Autodesk Inventor part; units mm, degrees
ref_plane "Work Plane1" through (-14.5, -35, 0) normal (0, -1, 0) x (1, 0, 0)
ref_plane "Work Plane4" through (-14.5, -35, 0) normal (-1, 0, 0) x (0, 0, 1)
ref_plane "YZ Plane" through (0, 0, 0) normal (1, 0, 0) x (0, 1, 0)
ref_plane "Work Plane1" through (-14.5, -35, 0) normal (0, -1, 0) x (1, 0, 0)
sketch "Sketch2" plane through (-14.5, -35, 0) normal (0, -1, 0) x (1, 0, 0)
  line L0 (4.3469, 0) -> (4.3469, 20)
  line L1 (7.596, 20) -> (7.4184, 20)
  line L2 (4.3469, 20) -> (7.596, 20)
  arc A0 (7.596, 20) -> (29, 8.6937) centre (18.17, 14.1045) ccw
  line L3 (4.3469, 0) -> (18.3998, 0)
  arc A1 (18.3998, 0) -> (29, 8.6937) centre (18.9461, 10.1431) ccw
  point P0 (14.5, 0)
  point P1 (5, 0)
  point P2 (18.2531, 1.9984)
extrude "Extrusion1" add sketch "Sketch2" against normal blind 15
ref_plane "Work Plane4" through (-14.5, -35, 0) normal (-1, 0, 0) x (0, 0, 1)
sketch "Sketch3" plane through (-14.5, -35, 0) normal (-1, 0, 0) x (0, 0, 1)
  line L0 (20, 0) -> (20, 70)
  line L1 (0, 0) -> (0, 21)
  line L2 (20, 70) -> (0, 70)
  line L3 (0, 70) -> (0, 0)
  line L4 (0, 0) -> (20, 0)
  line L5 (20, 0) -> (20, 70)
  point P0 (0, 35)
extrude "Extrusion2" add sketch "Sketch3" against normal blind 5.5
mirror "Mirror3" about plane through (0, 0, 0) normal (0, 1, 0) of "Extrusion1"
sketch "Sketch4" plane through (-9, -35, 0) normal (1, 0, 0) x (0, 0, -1)
  line L0 (-20, 15) -> (-1.9981, 15)
  line L1 (-12.7438, 15) -> (-12.7438, 55)
  line L2 (0, 55) -> (-20, 55)
  line L3 (-12.7438, 35) -> (-17.7089, 35)
  circle A0 centre (-12.7438, 35) radius 1.5
  point P0 (0, 35)
  point P1 (-8.6937, 15)
  dimension "d4" = 3
extrude "Extrusion3" cut sketch "Sketch4" against normal blind 10.375
sketch "Sketch5" plane through (-14.5, -35, 0) normal (-1, 0, 0) x (0, 0, 1)
  line L0 (20, 70) -> (0, 70)
  line L1 (0, 0) -> (20, 0)
  line L2 (20, 70) -> (0, 70)
  line L3 (0, 70) -> (0, 0)
  line L4 (0, 0) -> (20, 0)
  line L5 (20, 0) -> (20, 70)
  point P0 (0, 35)
extrude "Extrusion4" cut sketch "Sketch5" against normal blind 2
sketch "Sketch7" plane through (-14.5, -35, 0) normal (0, -1, 0) x (1, 0, 0)
  line L0 (7.596, 20) -> (2, 20)
  line L1 (2, 20) -> (2, 0)
  line L2 (2, 20) -> (2, 0)
  arc A0 (18.3998, 0) -> (29, 8.6937) centre (18.9461, 10.1431) ccw
  line L3 (5.5, 20) -> (7.596, 20)
  arc A1 (7.596, 20) -> (29, 8.6937) centre (18.17, 14.1045) ccw
  arc A2 (7.596, 20) -> (29, 8.6937) centre (18.17, 14.1045) ccw
  arc A3 (19.4924, 0) -> (29, 8.6937) centre (18.9461, 10.1431) ccw
  line L4 (2, 20) -> (7.596, 20)
  line L5 (2, 0) -> (18.3998, 0)
  line L6 (2, 0) -> (18.3998, 0)
  point P0 (14.5, 0)
extrude "Extrusion5" cut sketch "Sketch7" against normal blind 6
sketch "Sketch8" plane through (-12.5, 35, 0) normal (0, 1, 0) x (1, 0, 0)
  line L0 (3.5, -20) -> (5.596, -20)
  line L1 (0, 0) -> (0, -20)
  line L2 (5.596, -20) -> (0, -20)
  line L3 (0, -20) -> (0, 0)
  arc A0 (27, -8.6937) -> (16.3998, 0) centre (16.9461, -10.1431) ccw
  line L4 (0, 0) -> (16.3998, 0)
  arc A1 (27, -8.6937) -> (5.596, -20) centre (16.17, -14.1045) ccw
  arc A2 (27, -8.6937) -> (5.596, -20) centre (16.17, -14.1045) ccw
  arc A3 (27, -8.6937) -> (16.3998, 0) centre (16.9461, -10.1431) ccw
  point P0 (12.5, 0)
extrude "Extrusion6" cut sketch "Sketch8" against normal blind 6
properties part number "Speed Champ"
Design review of the part built by this model. Coordinates are the model's own, in mm. A direction names the side the tool comes from. Coordinates: 2 decimals unless noted, no trailing zeros. Loops run counter-clockwise (first coordinate to the right, second up) from the corner with the lowest first, then second, coordinate; pieces in that order, holes last. Notation, with made-up numbers: (80, -25.5) - (121, -25.5) arc R9 cw to (121, -9.5) - close; hole circle Ø1 at (62.5, 78.5). An arc over 180 degrees is marked (long way). Use CSV: the item, a comma, the result in double quotes. Start each with the question number.
1) The part is to be moulded in two halves that separate along Y. For faces 1 (the cylindrical face through (10.969, 24.563, 2.356)), 2 (the flat face through (-6, -29, 6)), 3 (the cylindrical face through (-10.726, -0.575, 11.358)), say which applies: +Y half, -Y half, draft (parallel to the pull), parting line (faces both ways), or undercut.
2) Consider section D-D on z = 16.5. Write out the cut boundary in (x, y).
3) Wall thickness on L1, parallel to Z at x = -11, y = 0; L2, parallel to X at y = -17.5, z = 7.75; L3, parallel to Z at x = -9.5, y = 19.5: over which ranges is each line inside the solid? List them lowest first. Write a range as from..to.
4) For pin 1 Ø10 at (y, z) = (-1, 7) entering from +X, flat-tipped, find the tip position at first contact; note if it passes through.
5) Consider section A-A on y = 0. Write out the cut boundary in (x, z), then the cut area to 3 significant figures.
6) Consider section C-C on z = 12.5. Write out the cut boundary in (x, y).
7) Tool access review of faces 4 (the flat face through (-10, 0, 20)), 5 (the flat face through (-3, -20, 3)): name each direction out of +Z, -Z, +X, -X, +Y, -Y from which nothing blocks a thin tool from reaching the whole face with its end or side.
8) Consider section B-B on x = 3. Write out the cut boundary in (y, z).
Geometry says:
1,face 1,"draft"
1,face 2,"-Y half"
1,face 3,"undercut"
2,outline,"(-12.5, -29) - (-8.2, -29) - (-8.2, -20) - (-9, -20) - (-9, 20) - (-8.2, 20) - (-8.2, 29) - (-12.5, 29) - close"
3,L1,"0..11.24, 14.24..20"
3,L2,"-12.5..-9"
3,L3,"0..20"
4,pin 1,"x = -9"
5,outline,"(-12.5, 0) - (-9, 0) - (-9, 11.24) - (-12.5, 11.24) - close; (-12.5, 14.24) - (-9, 14.24) - (-9, 20) - (-12.5, 20) - close"
5,area,"59.5 mm^2"
6,outline,"(-12.5, -29) - (-8.33, -29) - (-8.33, -20) - (-9, -20) - (-9, -1.48) - (-12.5, -1.48) - close; (-12.5, 1.48) - (-9, 1.48) - (-9, 20) - (-8.33, 20) - (-8.33, 29) - (-12.5, 29) - close"
7,face 4,"+Z, +X, -X, +Y, -Y"
7,face 5,"+Z, -Z, +X"
8,outline,"(-29, 0) - (-20, 0) - (-20, 2.02) - (-29, 2.02) - close; (20, 0) - (29, 0) - (29, 2.02) - (20, 2.02) - close"
